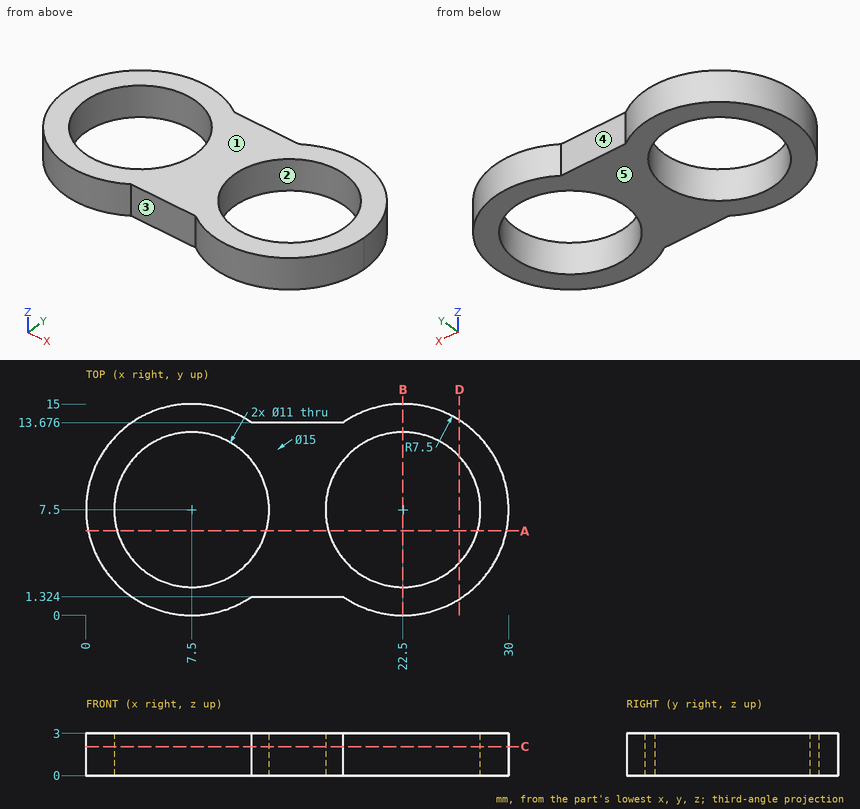
The figure shows three views and two pictorial views of one solid part (mm, origin at its lowest corner). Answer the questions. A direction names the side the tool comes from. Round coordinates to 2 decimals unless told otherwise and drop trailing zeros. Write each loop counter-clockwise with the first axis right and the second up, starting at its lowest first coordinate (ties: lowest second). Pieces come first, ordered by that corner, then holes. Notation, with made-up numbers: M -28.5,74 L 22.5,74 A18 cw 22.5,85 Z; hole C 52.25,53.5 d6. An arc over 180 degrees is marked long. Use a Markdown table: item, result.
1) The part is cut by section C-C on z = 2.05. Give the vertices of the cut face in (x, y).
Taken from the geometry:
| item | result |
|---|---|
| outline | M 11.76,1.32 L 18.24,1.32 A7.5 ccw long 18.24,13.68 L 11.76,13.68 A7.5 ccw long Z; hole C 7.5,7.5 d11; hole C 22.5,7.5 d11 |
2) The part is cut by section D-D on x = 26.5. Give the vertices of the cut face in (y, z) (1 decimal), plus the area to 3 significant figures.
Taken from the geometry:
| item | result |
|---|---|
| outline | M 1.2,0 L 3.7,0 L 3.7,3 L 1.2,3 Z; M 11.3,0 L 13.8,0 L 13.8,3 L 11.3,3 Z |
| area | 15.4 mm2 |
3) The part is cut by section A-A on y = 6. Give the vertices of the cut face in (x, z).
Taken from the geometry:
| item | result |
|---|---|
| outline | M 0.15,0 L 2.21,0 L 2.21,3 L 0.15,3 Z; M 12.79,0 L 17.21,0 L 17.21,3 L 12.79,3 Z; M 27.79,0 L 29.85,0 L 29.85,3 L 27.79,3 Z |
4) Which of the six approach directions +Z, -Z, +X, -X, +Y, -Y give full straight-line access (tool end or side, diameter ignored) to the marked faces 3, 4 and 5?
Taken from the geometry:
| item | result |
|---|---|
| face 3 | +Z, -Z, -Y |
| face 4 | +Z, -Z, +Y |
| face 5 | -Z, +X, -X, +Y, -Y |
5) Flat-ended cylindrical pins translate along their axes: pin 1 (0.9 mm diameter, centred on x = 16, z = 1, fed in from -Y); pin 2 (4 mm diameter, centred on x = 21, y = 2.5, fed in from -Z). Find the tip coordinate at first contact, or state that the pin passes through.
Taken from the geometry:
| item | result |
|---|---|
| pin 1 | stops at y = 1.32 |
| pin 2 | stops at z = 0 |
6) Consider line 1 (X direction, y = 7.5, z = 0.5); line 2 (X direction, y = 12, z = 2.45); line 3 (Y direction, x = 22.5, z = 1.4). Determine where each line is inside the solid, lowest interval first. Write a range as [from, to].
Taken from the geometry:
| item | result |
|---|---|
| line 1 | x = [0, 2], [13, 17], [28, 30] |
| line 2 | x = [1.5, 4.34], [10.66, 19.34], [25.66, 28.5] |
| line 3 | y = [0, 2], [13, 15] |
7) Determine the mould class of the marked faces 1 and 2 for opening direction X: pulls with the +X half, pulls with the -X half, needs draft (parallel to the pull), parting line crosses it, or undercut.
Taken from the geometry:
| item | result |
|---|---|
| face 1 | needs draft |
| face 2 | undercut |
8) The part is cut by section B-B on x = 22.5. Give the vertices of the cut face in (y, z).
Taken from the geometry:
| item | result |
|---|---|
| outline | M 0,0 L 2,0 L 2,3 L 0,3 Z; M 13,0 L 15,0 L 15,3 L 13,3 Z |
